from build123d import *

# Parameters (mm, degrees)
SKETCH1_R           = 1.5
BOSS_EXTRUDE1_DEPTH = 1.75
BOSS_EXTRUDE6_DEPTH = 1
BOSS_EXTRUDE7_DEPTH = 0.5
CUT_EXTRUDE1_REACH  = 3.5
SKETCH7_R           = 0.25


with BuildPart() as part:
    # Sketch1 → Boss-Extrude1 (new body)
    with BuildSketch(Plane(origin=(0, 0, 0), x_dir=(1, 0, 0), z_dir=(0, 1, 0))):
        with BuildLine():
            Line((-16, 18), (16, 18))
            ThreePointArc((16, 18), (17.414213562, 17.414213562), (18, 16))
            Line((18, 16), (18, -16))
            ThreePointArc((18, -16), (17.414213562, -17.414213562), (16, -18))
            Line((16, -18), (-16, -18))
            ThreePointArc((-16, -18), (-17.414213562, -17.414213562), (-18, -16))
            Line((-18, -16), (-18, 16))
            ThreePointArc((-18, 16), (-17.414213562, 17.414213562), (-16, 18))
        make_face()
        with Locations((-15.25, 15.25)):
            Circle(SKETCH1_R, mode=Mode.SUBTRACT)
        with Locations((15.25, 15.25)):
            Circle(SKETCH1_R, mode=Mode.SUBTRACT)
        with Locations((-15.25, -15.25)):
            Circle(SKETCH1_R, mode=Mode.SUBTRACT)
        with Locations((15.25, -15.25)):
            Circle(SKETCH1_R, mode=Mode.SUBTRACT)
    extrude(amount=BOSS_EXTRUDE1_DEPTH)

    # Sketch2 → Boss-Extrude6 (add)
    with BuildSketch(Plane.XY.offset(18)):
        with BuildLine():
            Line((2.843456523, 4.116656207), (5.398697456, 4.116656207))
            ThreePointArc((5.398697456, 4.116656207), (5.540118812, 4.058077564), (5.598697456, 3.916656207))
            Line((5.598697456, 3.916656207), (5.598697456, 3.555649959))
            ThreePointArc((5.598697456, 3.555649959), (5.6572761, 3.414228602), (5.798697456, 3.355649959))
            Line((5.798697456, 3.355649959), (5.933688948, 3.355649959))
            ThreePointArc((5.933688948, 3.355649959), (6.075110304, 3.297071315), (6.133688948, 3.155649959))
            Line((6.133688948, 3.155649959), (6.133688948, 1.75))
            Line((6.133688948, 1.75), (2.133688948, 1.75))
            Line((2.133688948, 1.75), (2.133688948, 3.155649959))
            ThreePointArc((2.133688948, 3.155649959), (2.192267592, 3.297071315), (2.333688948, 3.355649959))
            Line((2.333688948, 3.355649959), (2.443456523, 3.355649959))
            ThreePointArc((2.443456523, 3.355649959), (2.58487788, 3.414228602), (2.643456523, 3.555649959))
            Line((2.643456523, 3.555649959), (2.643456523, 3.916656207))
            ThreePointArc((2.643456523, 3.916656207), (2.702035167, 4.058077564), (2.843456523, 4.116656207))
        make_face()
        with BuildLine():
            Line((2.843456523, 4.016656207), (5.398697456, 4.016656207))
            ThreePointArc((5.398697456, 4.016656207), (5.469408134, 3.987366886), (5.498697456, 3.916656207))
            Line((5.498697456, 3.916656207), (5.498697456, 3.555649959))
            ThreePointArc((5.498697456, 3.555649959), (5.586565422, 3.343517924), (5.798697456, 3.255649959))
            Line((5.798697456, 3.255649959), (5.933688948, 3.255649959))
            ThreePointArc((5.933688948, 3.255649959), (6.004399626, 3.226360637), (6.033688948, 3.155649959))
            Line((6.033688948, 3.155649959), (6.033688948, 1.85))
            Line((6.033688948, 1.85), (2.233688948, 1.85))
            Line((2.233688948, 1.85), (2.233688948, 3.155649959))
            ThreePointArc((2.233688948, 3.155649959), (2.26297827, 3.226360637), (2.333688948, 3.255649959))
            Line((2.333688948, 3.255649959), (2.443456523, 3.255649959))
            ThreePointArc((2.443456523, 3.255649959), (2.655588558, 3.343517924), (2.743456523, 3.555649959))
            Line((2.743456523, 3.555649959), (2.743456523, 3.916656207))
            ThreePointArc((2.743456523, 3.916656207), (2.772745845, 3.987366886), (2.843456523, 4.016656207))
        make_face(mode=Mode.SUBTRACT)
    extrude(amount=-BOSS_EXTRUDE6_DEPTH)

    # Sketch6 → Boss-Extrude7 (add)
    with BuildSketch(Plane(origin=(0, 0, 17), x_dir=(-1, 0, 0), z_dir=(0, 0, -1))):
        with BuildLine():
            Line((-5.598697456, 3.916656207), (-5.598697456, 3.555649959))
            ThreePointArc((-5.598697456, 3.555649959), (-5.6572761, 3.414228602), (-5.798697456, 3.355649959))
            Line((-5.798697456, 3.355649959), (-5.933688948, 3.355649959))
            ThreePointArc((-5.933688948, 3.355649959), (-6.075110304, 3.297071315), (-6.133688948, 3.155649959))
            Line((-6.133688948, 3.155649959), (-6.133688948, 1.75))
            Line((-6.133688948, 1.75), (-2.133688948, 1.75))
            Line((-2.133688948, 1.75), (-2.133688948, 3.155649959))
            ThreePointArc((-2.133688948, 3.155649959), (-2.192267592, 3.297071315), (-2.333688948, 3.355649959))
            Line((-2.333688948, 3.355649959), (-2.443456523, 3.355649959))
            ThreePointArc((-2.443456523, 3.355649959), (-2.58487788, 3.414228602), (-2.643456523, 3.555649959))
            Line((-2.643456523, 3.555649959), (-2.643456523, 3.916656207))
            ThreePointArc((-2.643456523, 3.916656207), (-2.702035167, 4.058077564), (-2.843456523, 4.116656207))
            Line((-2.843456523, 4.116656207), (-5.398697456, 4.116656207))
            ThreePointArc((-5.398697456, 4.116656207), (-5.540118812, 4.058077564), (-5.598697456, 3.916656207))
        make_face()
    extrude(amount=BOSS_EXTRUDE7_DEPTH)

    # Sketch7 → Cut-Extrude1 (cut, up to next)
    with BuildSketch(Plane(origin=(0, 0, 16.5), x_dir=(-1, 0, 0), z_dir=(0, 0, -1)), mode=Mode.PRIVATE) as cut_extrude1_sk1:
        with Locations((-4.878111957, 3.016893087)):
            Circle(SKETCH7_R)
    cut_extrude1_tool1 = extrude(cut_extrude1_sk1.sketch, amount=-CUT_EXTRUDE1_REACH, mode=Mode.PRIVATE) & part.part
    add(cut_extrude1_tool1.solids().sort_by_distance((4.878112, 3.016893, 16.5))[0], mode=Mode.SUBTRACT)
    # Sketch7 → Cut-Extrude1 (cut, up to next)
    with BuildSketch(Plane(origin=(0, 0, 16.5), x_dir=(-1, 0, 0), z_dir=(0, 0, -1)), mode=Mode.PRIVATE) as cut_extrude1_sk2:
        with Locations((-4.078118838, 3.013574967)):
            Circle(SKETCH7_R)
    cut_extrude1_tool2 = extrude(cut_extrude1_sk2.sketch, amount=-CUT_EXTRUDE1_REACH, mode=Mode.PRIVATE) & part.part
    add(cut_extrude1_tool2.solids().sort_by_distance((4.078119, 3.013575, 16.5))[0], mode=Mode.SUBTRACT)
    # Sketch7 → Cut-Extrude1 (cut, up to next)
    with BuildSketch(Plane(origin=(0, 0, 16.5), x_dir=(-1, 0, 0), z_dir=(0, 0, -1)), mode=Mode.PRIVATE) as cut_extrude1_sk3:
        with Locations((-3.278127018, 3.00995723)):
            Circle(SKETCH7_R)
    cut_extrude1_tool3 = extrude(cut_extrude1_sk3.sketch, amount=-CUT_EXTRUDE1_REACH, mode=Mode.PRIVATE) & part.part
    add(cut_extrude1_tool3.solids().sort_by_distance((3.278127, 3.009957, 16.5))[0], mode=Mode.SUBTRACT)


solid = part.part
Check sheet for the modelled part. Datum: model origin and axes. Units: mm. A direction names the side the tool comes from. Round coordinates to 2 decimals unless told otherwise and drop trailing zeros. Write each loop counter-clockwise with the first axis right and the second up, starting at its lowest first coordinate (ties: lowest second). Pieces come first, ordered by that corner, then holes. Notation, with made-up numbers: (29.25, 84.25) -> (55.25, 84.25) arc R18 ccw to (55.25, 115.25) -> close; hole circle Ø5 at (34.5, -2). An arc over 180 degrees is marked (long way). Answer as CSV lines item,"result". Start each with the question number.
1) Section check A-A on x = -15.25. Enter the section's corners in (y, z).
2) Section check B-B on z = 15.25. Enter the section's corners in (x, y).
3) Section check C-C on x = 1. Enter the section's corners in (y, z), and give its area (3 significant figures).
4) Release check for a two-part mould opening along Y. For faces 4 (the flat face through (4.2, 1.85, 17.5)), 5 (the flat face through (0, 1, -18)), 6 (the flat face through (0, 0, 0)) record: pulls with the +Y half, pulls with the -Y half, needs draft (parallel to the pull), parting line crosses it, or undercut.
5) Go/stop test with flat-tipped pins: P1, Ø3.5, axis at x = -15.25, z = -15.25, coming from the +Y side; P2, Ø0.5, axis at y = 2.5, z = 17.5, coming from the -X side. Record where each tip stops, or that it passes through.
6) Tool access check on faces 1 (the flat face through (-18, 1, 0)), 2 (the flat face through (4, 2, 16.5)), 3 (the flat face through (4.2, 2.5, 17)). Record the directions out of +Z, -Z, +X, -X, +Y, -Y that give a thin tool (end or side, any length) a straight path to the whole face; none if there is none.
7) Material ranges on line 1 (Z direction, x = 15.25, y = 1.1); line 2 (Z direction, x = 14, y = 1.1), recorded low to high. Write a range as from..to.
Found:
1,outline,"(0, -18) -> (1.75, -18) -> (1.75, -16.75) -> (0, -16.75) -> close; (0, -13.75) -> (1.75, -13.75) -> (1.75, 13.75) -> (0, 13.75) -> close; (0, 16.75) -> (1.75, 16.75) -> (1.75, 18) -> (0, 18) -> close"
2,outline,"(-18, 0) -> (-16.75, 0) -> (-16.75, 1.75) -> (-18, 1.75) -> close; (-13.75, 0) -> (13.75, 0) -> (13.75, 1.75) -> (-13.75, 1.75) -> close; (16.75, 0) -> (18, 0) -> (18, 1.75) -> (16.75, 1.75) -> close"
3,outline,"(0, -18) -> (1.75, -18) -> (1.75, 18) -> (0, 18) -> close"
3,area,"63.0 mm^2"
4,face 4,"undercut"
4,face 5,"needs draft"
4,face 6,"pulls with the -Y half"
5,P1,"stops at y = 1.75"
5,P2,"stops at x = 2.13"
6,face 1,"+Z, -Z, -X, +Y, -Y"
6,face 2,"-Z, +X, -X, +Y"
6,face 3,"+Z"
7,line 1,"z = -18..-16.75, -13.75..13.75, 16.75..18"
7,line 2,"z = -18..-16.08, -14.42..14.42, 16.08..18"
